Part model, mm, in its own coordinate system. Give positions to 0.01 mm unless a question says otherwise; leave off trailing zeros. Write each loop counter-clockwise with the first axis right and the second up, starting at its lowest first coordinate (ties: lowest second). Pieces come first, ordered by that corner, then holes. Notation, with made-up numbers: M -22,-23 L -12,-23 A9 cw -12,-16 Z; hole C -40,32.25 d11. An arc over 180 degrees is marked long. Answer as CSV lines item,"result". Start each with the question number.
1) Pin check, flat tips, straight feed: pin 1 Ø3 at (x, z) = (-3.5, 4) entering from +Y; pin 2 Ø4 at (x, z) = (2.5, 25.5) entering from -Y; pin 3 Ø6 at (y, z) = (3.5, 10) entering from -X. Stop position of each tip, or through.
2) Slice it at C-C, the plane y = 4. Give the cut face in (x, z) (3 decimals).
3) Wall check: line 1 along Z through (x, y) = (2.5, 0) (3 decimals); line 2 along Y through (x, z) = (-5, -36); line 3 along Y through (x, z) = (4.5, 23). Give the ranges that are in metal, low to high. Write a range as from..to.
4) Slice it at B-B, the plane z = 21. Give the cut face in (x, y) (3 decimals).
5) Slice it at A-A, the plane x = 2.75. Give the cut face in (y, z) (3 decimals), plus the area to 3 significant figures.
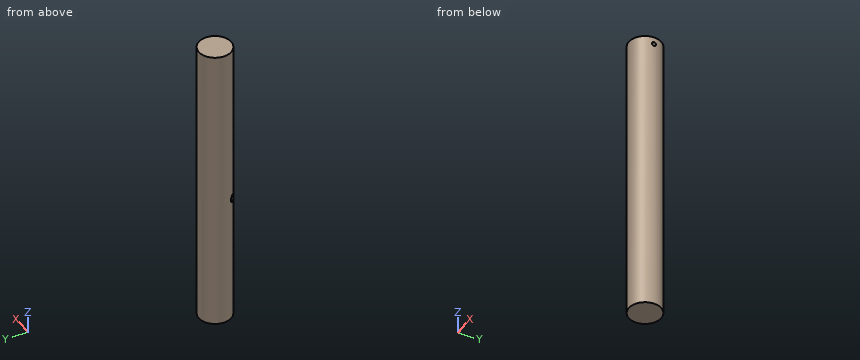
```python
from build123d import *

# Parameters (mm, degrees)
SKETCH1_R           = 3.81
BOSS_EXTRUDE1_DEPTH = 34.29
SCALE1_SCALE        = 1.5
SKETCH2_R           = 0.762
CUT_EXTRUDE1_DEPTH  = 53.066127905
SKETCH3_R           = 1.397
CUT_EXTRUDE2_DEPTH  = 53.066128026


with BuildPart() as part:
    # Sketch1 → Boss-Extrude1 (new, symmetric)
    with BuildSketch(Plane.XY):
        Circle(SKETCH1_R)
    extrude(amount=BOSS_EXTRUDE1_DEPTH, both=True)


with BuildPart() as part_1:
    # Scale1: scaled about (0, 0, 0)
    add(part.part.scale(SCALE1_SCALE))

    # Sketch2 → Cut-Extrude1 (cut, through all)
    with BuildSketch(Plane(origin=(0, 0, 0), x_dir=(0, 0, -1), z_dir=(1, 0, 0))):
        with Locations((-48.895, 0)):
            Circle(SKETCH2_R)
    extrude(amount=CUT_EXTRUDE1_DEPTH, mode=Mode.SUBTRACT)

    # Sketch3 → Cut-Extrude2 (cut, through all)
    with BuildSketch(Plane(origin=(0, 0, 0), x_dir=(-0.7071067811865476, 0.7071067811865476, 0), z_dir=(0.7071067811865476, 0.7071067811865476, 0))):
        with Locations((0, -5.715)):
            Circle(SKETCH3_R)
    extrude(amount=-CUT_EXTRUDE2_DEPTH, mode=Mode.SUBTRACT)


solid = part_1.part
```
Found:
1,pin 1,"y = 5.35"
1,pin 2,"y = -5.69"
1,pin 3,"x = -5.69"
2,outline,"M -4.082,-51.435 L 4.082,-51.435 L 4.082,51.435 L -4.082,51.435 Z"
3,line 1,"-51.435..48.133, 49.657..51.435"
3,line 2,"-2.77..2.77"
3,line 3,"-3.52..3.52"
4,outline,"C 0,0 d11.43"
5,outline,"M -5.01,-51.435 L 5.01,-51.435 L 5.01,51.435 L -5.01,51.435 Z; hole C 0,48.895 d1.524"
5,area,"1,030 mm²"
